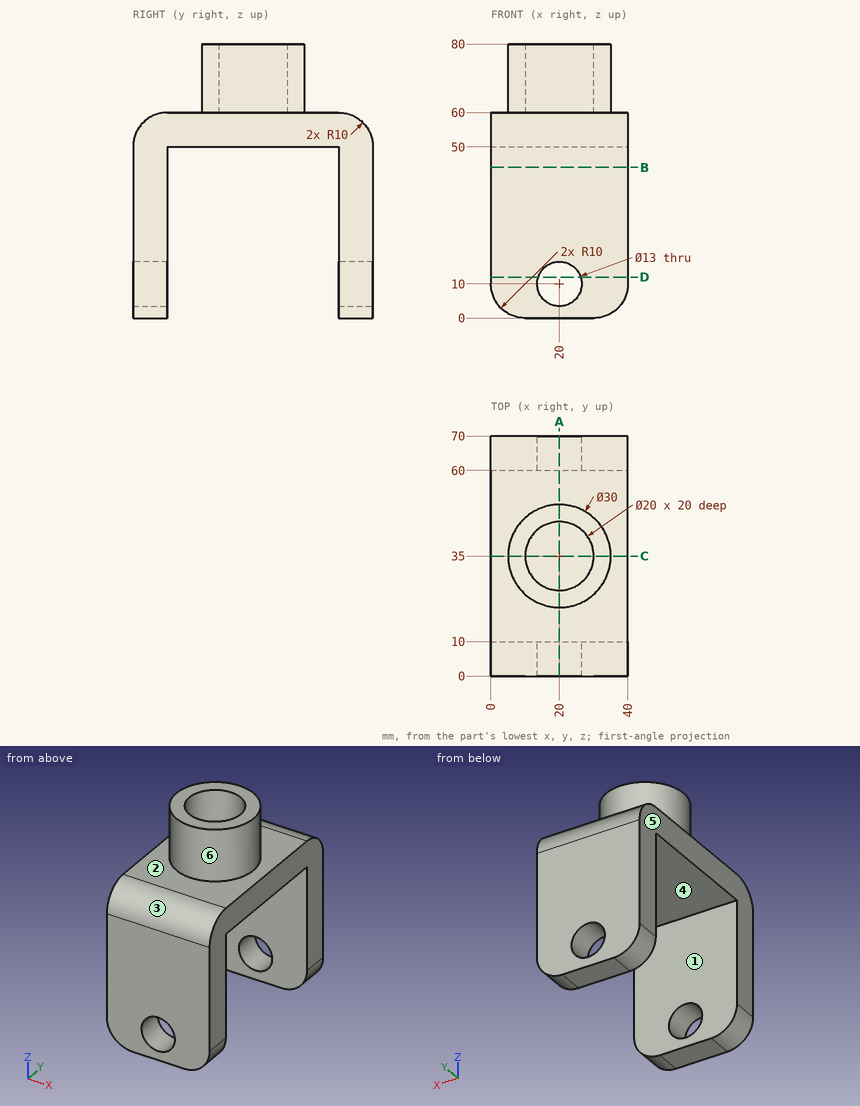
Part print with two shaded views. Sizes in mm from the minimum x, y, z corner. A direction names the side the tool comes from. Give positions to 0.01 mm unless a question says otherwise; leave off trailing zeros. Loops run counter-clockwise (first coordinate to the right, second up) from the corner with the lowest first, then second, coordinate; pieces in that order, holes last. Notation, with made-up numbers: (-31, 59) - (-2, 59) arc R17 ccw to (-2, 65) - close; hole circle Ø7 at (58.25, -9). An arc over 180 degrees is marked (long way). Put each result on its own line as item: value.
Q1. Slice it at A-A (x = 20). Give the cut face in (y, z), plus the area to 3 significant figures.
Filled in:
outline: (0, 0) - (10, 0) - (10, 3.5) - (0, 3.5) - close; (0, 16.5) - (10, 16.5) - (10, 50) - (60, 50) - (60, 16.5) - (70, 16.5) - (70, 50) arc R10 ccw to (60, 60) - (50, 60) - (50, 80) - (45, 80) - (45, 60) - (25, 60) - (25, 80) - (20, 80) - (20, 60) - (10, 60) arc R10 ccw to (0, 50) - close; (60, 0) - (70, 0) - (70, 3.5) - (60, 3.5) - close
area: 1,600 mm²
Q2. Probe line 1 along X through (y, z) = (65.25, 10); line 2 along Y through (x, z) = (20, 64.5); line 3 along Y through (x, z) = (15, 25). List the from-to ranges inside material, lowest first.
Filled in:
line 1: x = 0 to 13.5, 26.5 to 40
line 2: y = 20 to 25, 45 to 50
line 3: y = 0 to 10, 60 to 70
Q3. Slice it at B-B (z = 44). Give the cut face in (x, y), plus the area to 3 significant figures.
Filled in:
outline: (0, 0) - (40, 0) - (40, 10) - (0, 10) - close; (0, 60) - (40, 60) - (40, 70) - (0, 70) - close
area: 800 mm²
Q4. Slice it at D-D (z = 12). Give the cut face in (x, y).
Filled in:
outline: (0, 0) - (13.82, 0) - (13.82, 10) - (0, 10) - close; (0, 60) - (13.82, 60) - (13.82, 70) - (0, 70) - close; (26.18, 0) - (40, 0) - (40, 10) - (26.18, 10) - close; (26.18, 60) - (40, 60) - (40, 70) - (26.18, 70) - close
Q5. Flat gauge pins, fed straight in: pin 1 (4 mm diameter, centred on y = 29.5, z = 66, fed in from +X); pin 2 (2 mm diameter, centred on x = 16, y = 36.5, fed in from -Z); pin 3 (8 mm diameter, centred on y = 12.5, z = 67.5, fed in from -X); pin 4 (5 mm diameter, centred on x = 33.5, y = 57, fed in from +Z). Where does each tip first touch, or does it go through?
Filled in:
pin 1: stops at x = 34.59
pin 2: stops at z = 50
pin 3: passes through
pin 4: stops at z = 60
Q6. Tool access for the marked faces 4, 5 and 6: list every direction of +Z, -Z, +X, -X, +Y, -Y with a clear straight run to the whole face (end or side of a thin tool).
Filled in:
face 4: -Z, +X, -X
face 5: +Z, -Z, -X, +Y, -Y
face 6: +Z
Q7. Mould opens along Y. For the marked faces 1, 2 and 3 say: pulls with the +Y half, pulls with the -Y half, needs draft (parallel to the pull), parting line crosses it, or undercut.
Filled in:
face 1: undercut
face 2: needs draft
face 3: pulls with the -Y half
Q8. Slice it at C-C (y = 35). Give the cut face in (x, z), plus the area to 3 significant figures.
Filled in:
outline: (0, 50) - (40, 50) - (40, 60) - (35, 60) - (35, 80) - (30, 80) - (30, 60) - (10, 60) - (10, 80) - (5, 80) - (5, 60) - (0, 60) - close
area: 600 mm²
